Geometry: final body of the model. Coordinates: model frame, mm. A direction names the side the tool comes from. Round coordinates to 2 decimals unless told otherwise and drop trailing zeros. Write each loop counter-clockwise with the first axis right and the second up, starting at its lowest first coordinate (ties: lowest second). Pieces come first, ordered by that corner, then holes. Notation, with made-up numbers: (-26.5, 50.25) - (-9.5, 50.25) arc R31 ccw to (-9.5, 86.25) - close; hole circle Ø9 at (89.25, 6.25). An arc over 180 degrees is marked (long way). Use a Markdown table: item, result. Add a question column.
```python
from build123d import *

# Parameters (mm, degrees)
SKETCH_1_R      = 4
EXTRUDE_1_DEPTH = 12
SKETCH_2_R      = 6
EXTRUDE_2_DEPTH = 2
SKETCH_3_R      = 5.5
EXTRUDE_3_DEPTH = 4
CHAMFER_1_SIZE  = 0.5


with BuildPart() as part:
    # 草图1 → 凸台-拉伸1 (new body)
    with BuildSketch(Plane.XY):
        Circle(SKETCH_1_R)
    extrude(amount=EXTRUDE_1_DEPTH)

    # 草图2 → 凸台-拉伸2 (add)
    with BuildSketch(Plane(origin=(0, 0, 0), x_dir=(-1, 0, 0), z_dir=(0, 0, -1))):
        Circle(SKETCH_2_R)
    extrude(amount=EXTRUDE_2_DEPTH)

    # 草图3 → 凸台-拉伸3 (add)
    with BuildSketch(Plane(origin=(0, 0, -2), x_dir=(-1, 0, 0), z_dir=(0, 0, -1))):
        Circle(SKETCH_3_R)
    extrude(amount=EXTRUDE_3_DEPTH)

    # 草图4 → 旋转1 (revolve)
    with BuildSketch(Plane(origin=(0, 0, 0), x_dir=(1, 0, 0), z_dir=(0, 1, 0))):
        with BuildLine():
            Line((0, 8.2), (0, 0.2))
            ThreePointArc((0, 0.2), (4, 4.2), (0, 8.2))
        make_face()
    revolve(axis=Axis((0, 0, -9.405734293), (0, 0, 1)))

    # 倒角1
    chamfer_1_edges = [part.edges().sort_by_distance(p)[0] for p in [
        (-4, 0, 12),
    ]]
    chamfer(chamfer_1_edges, length=CHAMFER_1_SIZE)


solid = part.part
```
1) Material intervals for L1, parallel to Z at x = 4.25, y = 0.25; L2, parallel to X at y = 0.25, z = -1; L3, parallel to Y at x = -1.25, z = -1.75, sorted ascending. Write a range as from..to.
2) Section C-C, the plane z = -1. Return the cut outline in (x, y).
3) Section D-D, the plane y = -5. Return the cut outline in (x, z).
4) Set-up query: faces 1 (the flat face through (-4, 0, -6)), 2 (the cylindrical face through (6, 0, -1)), 3 (the cylindrical face through (-0.867, -3.905, 5.67)). Return all of +Z, -Z, +X, -X, +Y, -Y with unobstructed straight access to the full face (end or side cutting, diameter ignored); none if empty.
5) Pin query (flat end, axial travel): P1, Ø3, axis at x = 3, z = -0.5, coming from the -Y side; P2, Ø3.5, axis at x = -1, y = 3, coming from the -Z side; P3, Ø3, axis at x = 2, z = -1.5, coming from the +Y side. Return the tip coordinate at first contact, or that it passes through.
6) Section A-A, the plane y = 0. Return the cut outline in (x, z).
Output values:
| question | item | result |
|---|---|---|
| 1 | L1 | z = -6..0 |
| 1 | L2 | x = -5.99..5.99 |
| 1 | L3 | y = -5.87..5.87 |
| 2 | outline | circle Ø12 at (0, 0) |
| 3 | outline | (-3.32, -2) - (-2.29, -2) - (-2.29, -6) - (2.29, -6) - (2.29, -2) - (3.32, -2) - (3.32, 0) - (-3.32, 0) - close |
| 4 | face 1 | -Z |
| 4 | face 2 | +Z, -Z |
| 4 | face 3 | +Z |
| 5 | P1 | stops at y = -5.81 |
| 5 | P2 | stops at z = -7.94 |
| 5 | P3 | stops at y = 5.98 |
| 6 | outline | (-6, -2) - (-5.5, -2) - (-5.5, -6) - (-3.57, -6) arc R4 ccw to (3.57, -6) - (5.5, -6) - (5.5, -2) - (6, -2) - (6, 0) - (4, 0) - (4, 11.5) - (3.5, 12) - (-3.5, 12) - (-4, 11.5) - (-4, 0) - (-6, 0) - close |
